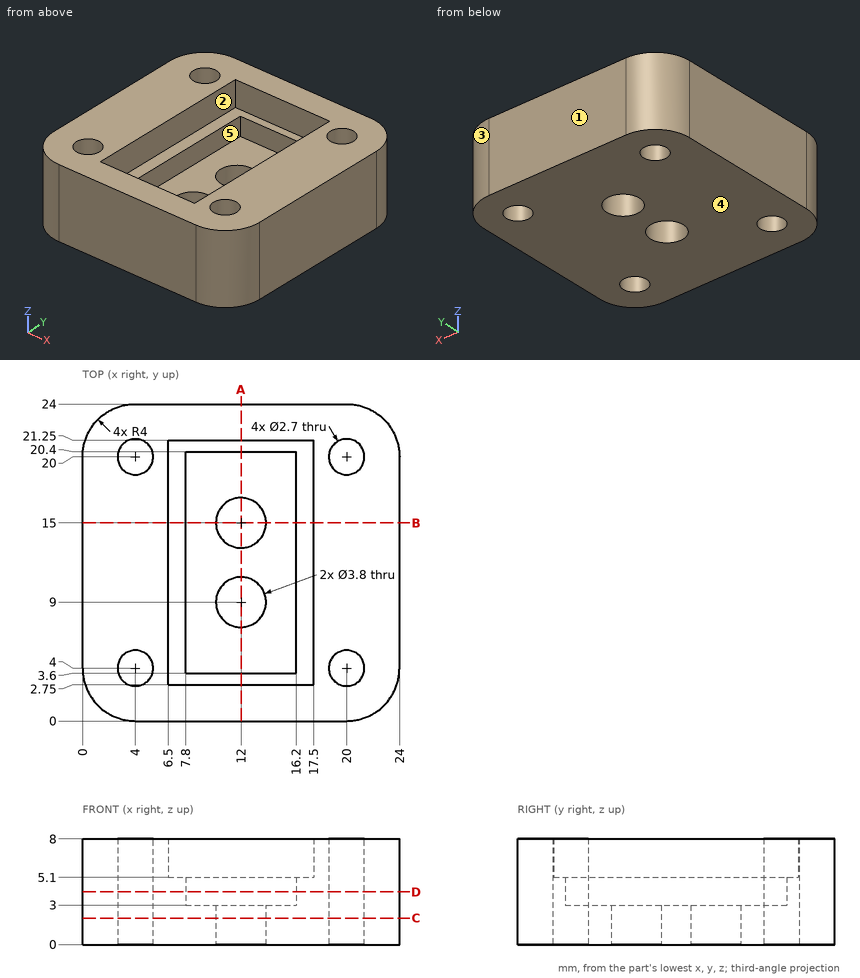
For this review, use the dimensioned drawing (mm, ordinates from the lowest corner) and the shaded views. A direction names the side the tool comes from. Coordinates: 2 decimals unless noted, no trailing zeros. Loops run counter-clockwise (first coordinate to the right, second up) from the corner with the lowest first, then second, coordinate; pieces in that order, holes last. Notation, with made-up numbers: (74, 8) - (91, 8) arc R10 ccw to (91, 12) - close; hole circle Ø6 at (9, 74.5). An arc over 180 degrees is marked (long way). Use one line per item in the form item = value. Start each with the question number.
1) To check wall thickness, follow probe 1 along Y at (x, z) = (4, 5.5); probe 2 along Y at (x, z) = (16.5, 5.5); probe 3 along X at (y, z) = (7.75, 7.5). State the ranges of each line that lie inside material, in increasing order. Write a range as from..to.
2) Draft analysis for pull direction X (two halves, no side actions). For the marked faces 1, 2 and 3, state which applies: released by +X, released by -X, zero draft, split by the parting line, or undercut.
3) Take a section at B-B (y = 15). State the section outline as (x, z) points.
4) Take a section at C-C (z = 2). State the section outline as (x, y) points, plus the area to 3 significant figures.
5) Take a section at D-D (z = 4). State the section outline as (x, y) points, plus the area to 3 significant figures.
6) For the marked faces 4 and 5, list the 3-axis set-ups (+Z, -Z, +X, -X, +Y, -Y) from which the entire face can be reached by the end or side of a thin tool; tool diameter is ignored.
7) Take a section at A-A (x = 12). State the section outline as (y, z) points, plus the area to 3 significant figures.
8) For pin 1 (5.5 mm diameter, centred on x = 13, y = 9.5, fed in from +Z), flat-tipped, find the tip position at first contact; note if it passes through.
From the geometry:
q1.probe_1 = 0..2.65, 5.35..18.65, 21.35..24
q1.probe_2 = 0..2.75, 21.25..24
q1.probe_3 = 0..6.5, 17.5..24
q2.face_1 = zero draft
q2.face_2 = undercut
q2.face_3 = released by +X
q3.outline = (0, 0) - (10.1, 0) - (10.1, 3) - (7.8, 3) - (7.8, 5.1) - (6.5, 5.1) - (6.5, 8) - (0, 8) - close; (13.9, 0) - (24, 0) - (24, 8) - (17.5, 8) - (17.5, 5.1) - (16.2, 5.1) - (16.2, 3) - (13.9, 3) - close
q4.outline = (0, 4) arc R4 ccw to (4, 0) - (20, 0) arc R4 ccw to (24, 4) - (24, 20) arc R4 ccw to (20, 24) - (4, 24) arc R4 ccw to (0, 20) - close; hole circle Ø2.7 at (4, 4); hole circle Ø2.7 at (4, 20); hole circle Ø3.8 at (12, 9); hole circle Ø3.8 at (12, 15); hole circle Ø2.7 at (20, 4); hole circle Ø2.7 at (20, 20)
q4.area = 517 mm2
q5.outline = (0, 4) arc R4 ccw to (4, 0) - (20, 0) arc R4 ccw to (24, 4) - (24, 20) arc R4 ccw to (20, 24) - (4, 24) arc R4 ccw to (0, 20) - close; hole circle Ø2.7 at (4, 4); hole circle Ø2.7 at (4, 20); hole (7.8, 3.6) - (16.2, 3.6) - (16.2, 20.4) - (7.8, 20.4) - close; hole circle Ø2.7 at (20, 4); hole circle Ø2.7 at (20, 20)
q5.area = 398 mm2
q6.face_4 = -Z, +X, -X, +Y, -Y
q6.face_5 = +Z
q7.outline = (0, 0) - (7.1, 0) - (7.1, 3) - (3.6, 3) - (3.6, 5.1) - (2.75, 5.1) - (2.75, 8) - (0, 8) - close; (10.9, 0) - (13.1, 0) - (13.1, 3) - (10.9, 3) - close; (16.9, 0) - (24, 0) - (24, 8) - (21.25, 8) - (21.25, 5.1) - (20.4, 5.1) - (20.4, 3) - (16.9, 3) - close
q7.area = 80.3 mm2
q8.pin_1 = 3
